Verification items for this drawing (mm, ordinates from the low corner). A direction names the side the tool comes from. Round coordinates to 2 decimals unless told otherwise and drop trailing zeros. Loops run counter-clockwise (first coordinate to the right, second up) from the corner with the lowest first, then second, coordinate; pieces in that order, holes last. Notation, with made-up numbers: (66, -25.75) -> (115, -25.75) arc R20 ccw to (115, 0.25) -> close; hole circle Ø1 at (-34.5, 20.5). An arc over 180 degrees is marked (long way). Use a Markdown table: item, result. Add a question column.
Q1. Gauge pin test, flat ends, axial feed: P1, Ø3, axis at y = 13.5, z = 27, coming from the -X side; P2, Ø10, axis at x = 13.5, y = 2, coming from the +Z side; P3, Ø12, axis at x = 29, z = 33, coming from the +Y side. Record the tip position at first contact, or that the pin passes through.
Q2. Sectioned sample at C-C, the plane z = 31.5. Enter the section's corners in (x, y), then the cut area to 3 significant figures.
Q3. Set-up check for the marked faces 1 and 2: record each of +Z, -Z, +X, -X, +Y, -Y from which the full face is reachable in a straight line by a thin tool's end or side.
Q4. Material ranges on L1, parallel to X at y = 1.5, z = 35; L2, parallel to Z at x = 37.5, y = 18, recorded low to high.
Q5. Sectioned sample at B-B, the plane x = 35. Enter the section's corners in (y, z), then the cut area to 3 significant figures.
Q6. Sectioned sample at A-A, the plane y = 4.75. Enter the section's corners in (x, z), then the cut area to 3 significant figures.
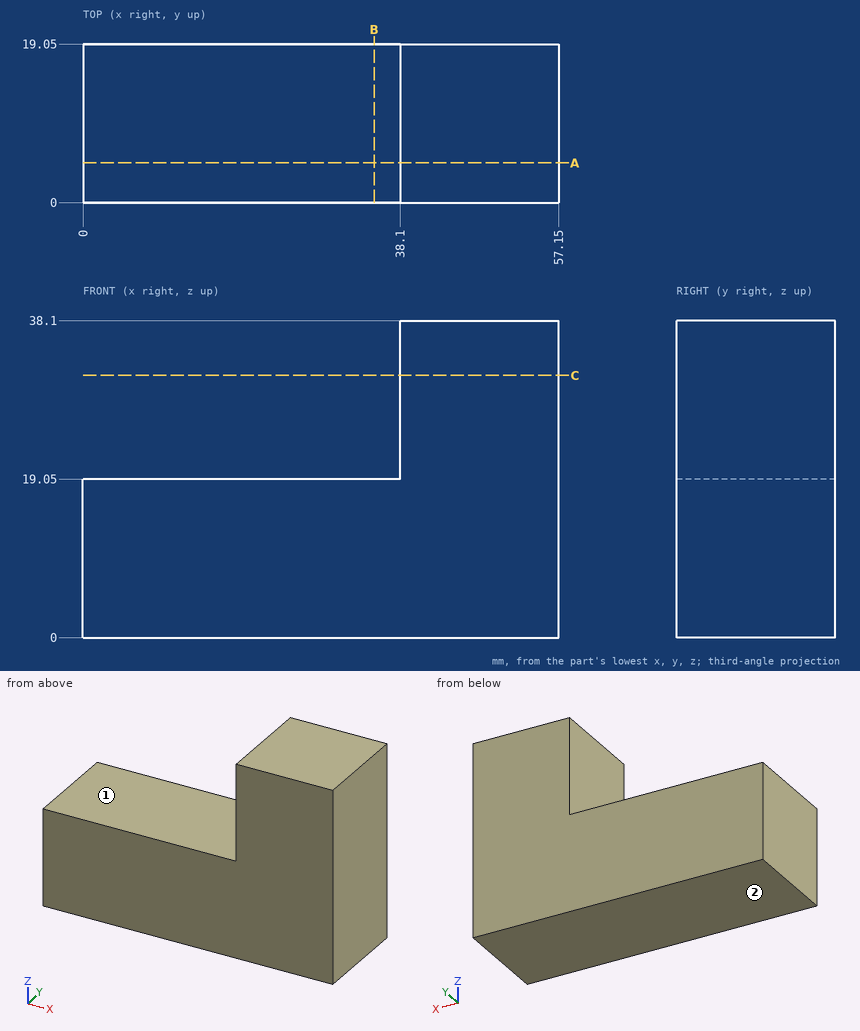
Values:
| question | item | result |
|---|---|---|
| 1 | P1 | x = 38.1 |
| 1 | P2 | z = 19.05 |
| 1 | P3 | through |
| 2 | outline | (38.1, 0) -> (57.15, 0) -> (57.15, 19.05) -> (38.1, 19.05) -> close |
| 2 | area | 363 mm^2 |
| 3 | face 1 | +Z, -X, +Y, -Y |
| 3 | face 2 | -Z, +X, -X, +Y, -Y |
| 4 | L1 | 38.1 to 57.15 |
| 4 | L2 | 0 to 19.05 |
| 5 | outline | (0, 0) -> (19.05, 0) -> (19.05, 19.05) -> (0, 19.05) -> close |
| 5 | area | 363 mm^2 |
| 6 | outline | (0, 0) -> (57.15, 0) -> (57.15, 38.1) -> (38.1, 38.1) -> (38.1, 19.05) -> (0, 19.05) -> close |
| 6 | area | 1,450 mm^2 |
